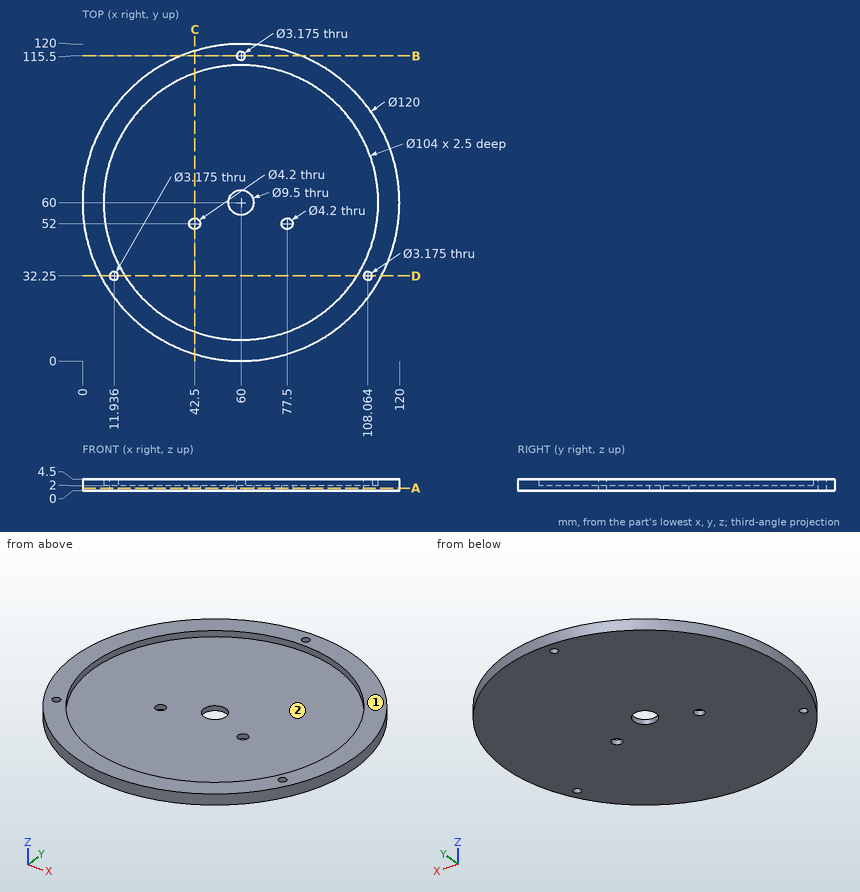
Check sheet for the drawn part. Datum: minimum x, y, z corner. Units: mm. Coordinates: 2 decimals unless noted, no trailing zeros. Loops run counter-clockwise (first coordinate to the right, second up) from the corner with the lowest first, then second, coordinate; pieces in that order, holes last. Notation, with made-up numbers: M 70,-37 L 81,-37 A17 cw 81,-7 Z; hole C 52.5,-24.75 d11. An arc over 180 degrees is marked long. Answer as a JSON object with one key per item and string values.
1. Sectioned sample at C-C on x = 42.5. Record the cut outline in (y, z), and give its area (3 significant figures).
Outcome:
{"outline": "M 2.61,0 L 49.9,0 L 49.9,2 L 11.03,2 L 11.03,4.5 L 2.61,4.5 Z; M 54.1,0 L 117.39,0 L 117.39,4.5 L 108.97,4.5 L 108.97,2 L 54.1,2 Z", "area": "263 mm²"}
2. Release check for a two-part mould opening along X. For the marked faces 1 and 2 record: pulls with the +X half, pulls with the -X half, needs draft (parallel to the pull), parting line crosses it, or undercut.
Outcome:
{"face 1": "needs draft", "face 2": "undercut"}
3. Depth check by flat-ended pin: P1, Ø5, axis at x = 77.5, y = 52, coming from the +Z side; P2, Ø2, axis at y = 52.5, z = 1.5, coming from the +X side; P3, Ø2, axis at x = 46.5, z = 1, coming from the +Y side. Enter the tip coordinate at first touch or a pass-through.
Outcome:
{"P1": "z = 2", "P2": "x = 119.65", "P3": "y = 118.68"}
4. Sectioned sample at A-A on z = 1.05. Count the separate pieces of the cut face and the enclosed holes in it, and give its area (3 significant figures).
Outcome:
{"separate pieces": "1", "enclosed holes": "6", "area": "11,200 mm²"}
5. Sectioned sample at B-B on y = 115.5. Record the cut outline in (x, z).
Outcome:
{"outline": "M 37.2,0 L 58.41,0 L 58.41,4.5 L 37.2,4.5 Z; M 61.59,0 L 82.8,0 L 82.8,4.5 L 61.59,4.5 Z"}
6. Scan lines: L1, parallel to Y at x = 60, z = 2.7; L2, parallel to Z at x = 98, y = 32.5; L3, parallel to Y at x = 71.5, z = 2.1. Record each from-to range of solid material in increasing order. Write a range as from..to.
Outcome:
{"L1": "0..8, 112..113.91, 117.09..120", "L2": "0..2", "L3": "1.11..9.29, 110.71..118.89"}
7. Sectioned sample at D-D on y = 32.25. Record the cut outline in (x, z).
Outcome:
{"outline": "M 6.8,0 L 10.35,0 L 10.35,4.5 L 6.8,4.5 Z; M 13.52,0 L 106.48,0 L 106.48,4.5 L 103.98,4.5 L 103.98,2 L 16.02,2 L 16.02,4.5 L 13.52,4.5 Z; M 109.65,0 L 113.2,0 L 113.2,4.5 L 109.65,4.5 Z"}
